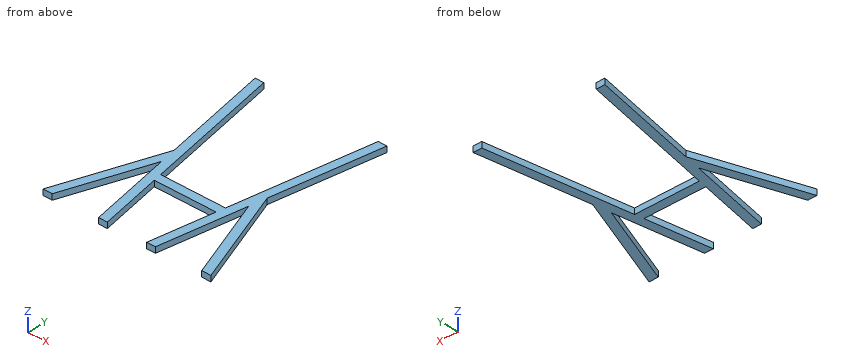
```python
from build123d import *

# Parameters (mm, degrees)
BOSS_EXTRU_1_DEPTH = 27
BOSS_EXTRU_2_DEPTH = 27


with BuildPart() as part:
    # Esquisse1 → Boss.-Extru.1 (new body)
    with BuildSketch(Plane.XY):
        Polygon((0, 0), (-173.648177667, 984.807753012), (-133.031113192, 984.807753012), (-18.530468053, 335.442325904), (281.469531947, 335.442325904), (395.970177086, 984.807753012), (436.587241561, 984.807753012), (262.939063894, 0), (222.321999419, 0), (274.416452719, 295.442325904), (-11.477388825, 295.442325904), (40.617064475, 0), align=None)
    extrude(amount=BOSS_EXTRU_1_DEPTH)

    # Esquisse2 → Boss.-Extru.2 (add)
    with BuildSketch(Plane.XY.offset(27)):
        Polygon((-69.948886071, 396.699845877), (-214.335821908, 0), (-256.902932807, 0), (-83.840740284, 475.484466118), align=None)
        Polygon((346.779804178, 475.484466118), (332.887949965, 396.699845877), (477.274885802, 0), (519.841996701, 0), align=None)
    extrude(amount=-BOSS_EXTRU_2_DEPTH)


solid = part.part
```
Geometry check sheet. Reference: the model listing, model coordinates, mm. Round coordinates to 2 decimals unless told otherwise and drop trailing zeros. Loops run counter-clockwise (first coordinate to the right, second up) from the corner with the lowest first, then second, coordinate; pieces in that order, holes last. Notation, with made-up numbers: (33, 61) - (82, 61) arc R8 cw to (82, 67) - close; hole circle Ø10 at (-22.5, -27). An arc over 180 degrees is marked (long way). Use a Markdown table: item, result.
Q1. Cross-section at D-D on x = 410. Record the cut outline in (y, z), plus the area to 3 significant figures.
Solutions:
| item | result |
|---|---|
| outline | (184.84, 0) - (301.79, 0) - (301.79, 27) - (184.84, 27) - close; (834.02, 0) - (984.81, 0) - (984.81, 27) - (834.02, 27) - close |
| area | 7,230 mm2 |
Q2. Cross-section at B-B on z = 16.75. Record the cut outline in (x, y), plus the area to 3 significant figures.
Solutions:
| item | result |
|---|---|
| outline | (-256.9, 0) - (-214.34, 0) - (-69.95, 396.7) - (0, 0) - (40.62, 0) - (-11.48, 295.44) - (274.42, 295.44) - (222.32, 0) - (262.94, 0) - (332.89, 396.7) - (477.27, 0) - (519.84, 0) - (346.78, 475.48) - (436.59, 984.81) - (395.97, 984.81) - (281.47, 335.44) - (-18.53, 335.44) - (-133.03, 984.81) - (-173.65, 984.81) - (-83.84, 475.48) - close |
| area | 129,000 mm2 |
Q3. Cross-section at A-A on y = 695. Record the cut outline in (x, z), plus the area to 3 significant figures.
Solutions:
| item | result |
|---|---|
| outline | (-122.55, 0) - (-81.93, 0) - (-81.93, 27) - (-122.55, 27) - close; (344.87, 0) - (385.49, 0) - (385.49, 27) - (344.87, 27) - close |
| area | 2,190 mm2 |
Q4. Cross-section at C-C on y = 196.5. Record the cut outline in (x, z), plus the area to 3 significant figures.
Solutions:
| item | result |
|---|---|
| outline | (-185.38, 0) - (-142.82, 0) - (-142.82, 27) - (-185.38, 27) - close; (-34.65, 0) - (5.97, 0) - (5.97, 27) - (-34.65, 27) - close; (256.97, 0) - (297.59, 0) - (297.59, 27) - (256.97, 27) - close; (405.75, 0) - (448.32, 0) - (448.32, 27) - (405.75, 27) - close |
| area | 4,490 mm2 |
Q5. Material ranges on line 1 (X direction, y = 83, z = 13.5); line 2 (X direction, y = 384, z = 2.25); line 3 (X direction, y = 309.5, z = 12.75), recorded low to high.
Solutions:
| item | result |
|---|---|
| line 1 | x = -226.69 to -184.13, -14.64 to 25.98, 236.96 to 277.57, 447.07 to 489.63 |
| line 2 | x = -117.14 to -74.57, -67.71 to -27.09, 290.03 to 330.65, 337.51 to 380.08 |
| line 3 | x = -144.25 to -101.69, -54.57 to 317.51, 364.63 to 407.19 |
Q6. Go/stop test with flat-tipped pins: P1, Ø1.5, axis at x = 42.5, z = 10.5, coming from the +Y side; P2, Ø4, axis at x = 71.5, z = 14, coming from the -Y side; P3, Ø6, axis at y = 733, z = 21, coming from the +X side. Record where each tip stops, or that it passes through.
Solutions:
| item | result |
|---|---|
| P1 | stops at y = 335.44 |
| P2 | stops at y = 295.44 |
| P3 | stops at x = 392.72 |
